Print and shaded views of the part. All mm, measured from the part's lowest x, y and z. A direction names the side the tool comes from. Round coordinates to 2 decimals unless told otherwise and drop trailing zeros. Write each loop counter-clockwise with the first axis right and the second up, starting at its lowest first coordinate (ties: lowest second). Pieces come first, ordered by that corner, then holes. Notation, with made-up numbers: M -19.5,-25.5 L 38.5,-25.5 A15 cw 38.5,-0.5 Z; hole C 39,65.5 d10. An arc over 180 degrees is marked long. Write item = value, one per line.
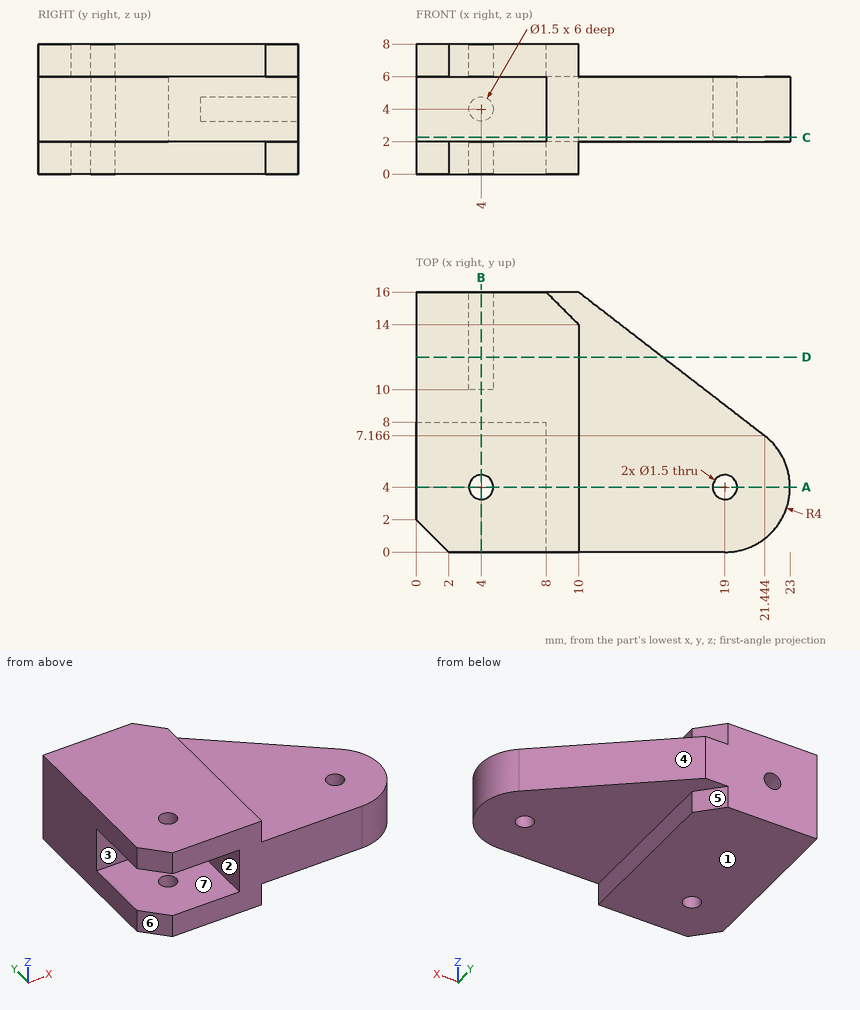
1. Band-saw the part on C-C (z = 2.25). List the corners of the cut face in (x, y).
Responses:
outline = M 0,8 L 8,8 L 8,0 L 19,0 A4 ccw 21.44,7.17 L 10,16 L 0,16 Z; hole C 19,4 d1.5
2. Band-saw the part on A-A (y = 4). List the corners of the cut face in (x, z).
Responses:
outline = M 0,0 L 3.25,0 L 3.25,2 L 0,2 Z; M 0,6 L 3.25,6 L 3.25,8 L 0,8 Z; M 4.75,0 L 10,0 L 10,2 L 18.25,2 L 18.25,6 L 10,6 L 10,8 L 4.75,8 L 4.75,6 L 8,6 L 8,2 L 4.75,2 Z; M 19.75,2 L 23,2 L 23,6 L 19.75,6 Z
3. Mould opens along Z. For the marked faces 1, 2, 3 and 4 say: pulls with the +Z half, pulls with the -Z half, needs draft (parallel to the pull), parting line crosses it, or undercut.
Responses:
face_1 = pulls with the -Z half
face_2 = undercut
face_3 = undercut
face_4 = needs draft
4. Tool access for the marked faces 5, 6 and 7: list every direction of +Z, -Z, +X, -X, +Y, -Y with a clear straight run to the whole face (end or side of a thin tool).
Responses:
face_5 = -Z, +X, +Y
face_6 = +Z, -Z, -X, -Y
face_7 = -X, -Y
5. Flat gauge pins, fed straight in: pin 1 (2.5 mm diameter, centred on x = 3.5, y = 4.5, fed in from +Z); pin 2 (0.6 mm diameter, centred on y = 6.5, z = 1, fed in from +X); pin 3 (1.5 mm diameter, centred on x = 20, z = 1.5, fed in from -Y); pin 4 (3 mm diameter, centred on y = 3.5, z = 4, fed in from -X). Where does each tip first touch, or does it go through?
Responses:
pin_1 = 8
pin_2 = 10
pin_3 = 0.02
pin_4 = 8
6. Probe probe 1 along Y at (x, z) = (4, 7.5); probe 2 along Z at (x, y) = (2.75, 5.75); probe 3 along Z at (x, y) = (4, 12.2). List the from-to ranges inside material, lowest first.
Responses:
probe_1 = 0 to 3.25, 4.75 to 16
probe_2 = 0 to 2, 6 to 8
probe_3 = 0 to 3.25, 4.75 to 8
7. Band-saw the part on D-D (y = 12). List the corners of the cut face in (x, z).
Responses:
outline = M 0,0 L 10,0 L 10,2 L 15.18,2 L 15.18,6 L 10,6 L 10,8 L 0,8 Z; hole C 4,4 d1.5
8. Band-saw the part on B-B (x = 4). List the corners of the cut face in (y, z).
Responses:
outline = M 0,0 L 3.25,0 L 3.25,2 L 0,2 Z; M 0,6 L 3.25,6 L 3.25,8 L 0,8 Z; M 4.75,0 L 16,0 L 16,3.25 L 10,3.25 L 10,4.75 L 16,4.75 L 16,8 L 4.75,8 L 4.75,6 L 8,6 L 8,2 L 4.75,2 Z
